The model under review builds one solid part; all positions refer to its coordinate system, in mm. A direction names the side the tool comes from. Coordinates: 2 decimals unless noted, no trailing zeros. Answer in a Markdown table with one row per item.
Autodesk Inventor part; units mm, degrees
ref_plane "YZ Plane" through (0, 0, 0) normal (1, 0, 0) x (0, 1, 0)
ref_plane "XZ Plane" through (0, 0, 0) normal (0, 1, 0) x (-1, 0, 0)
ref_plane "XY Plane" through (0, 0, 0) normal (0, 0, 1) x (1, 0, 0)
sketch "Sketch1" plane through (0, 0, 0) normal (0, 0, 1) x (1, 0, 0)
  line L0 (0, 0) -> (0, 24)
  line L1 (0, 24) -> (25, 24)
  line L2 (25, 24) -> (25, 4)
  line L3 (25, 4) -> (20, 4)
  line L4 (20, 4) -> (20, 0)
  line L5 (20, 0) -> (0, 0)
  line L6 (0, -4.8611) -> (0, 32.7303) construction
  dimension "d0" = 25
  dimension "d1" = 20
  dimension "d2" = 4
  dimension "d4" = 5
revolve "Revolution1" add sketch "Sketch1" angle 360 about axis through (0, -4.8611, 0) along (0, 1, 0)
sketch "Sketch9" plane through (0, 0, 0) normal (1, 0, 0) x (0, 1, 0)
  line L0 (0, 0) -> (-39.5663, 0) construction
  line L1 (4.5, -25) -> (5.5, -25)
  line L2 (5.5, -25) -> (5.5, -72.5)
  line L3 (5.5, -72.5) -> (4.5, -72.5)
  line L4 (4.5, -72.5) -> (4.5, -25)
  line L5 (0, -20) -> (0, 20)
  dimension "d28" = 1
  dimension "d29" = 25
  dimension "d30" = 4.5
  dimension "d31" = 47.5
coil "Coil1" sketch "Sketch9" operation add axis through (0, 0, 0) along (0, 1, 0) pitch 226 turns 0.077434 hand right
pattern_circular "Circular Pattern1" count 7 over 360 about axis through (0, 14, 0) along (0, 1, 0) of "Coil1"
equation "\"BendRadius\" = Thickness"
equation "\"BendReliefWidth\" = Thickness"
equation "\"BendReliefDepth\" = 0.5 * Thickness"
equation "\"CornerReliefSize\" = 4 * Thickness"
equation "\"MinimumRemnant\" = 2 * Thickness"
equation "\"TransitionRadius\" = BendRadius"
equation "\"JacobiRadiusSize\" = BendRadius"
equation "\"GapSize\" = Thickness"
properties part number "Ventoinha"
(1) Take a section at A-A (z = -36.5). State how many separate pieces and enclosed holes the cut face has, then the cut area to 3 significant figures.
Report:
| item | result |
|---|---|
| separate pieces | 3 |
| enclosed holes | 0 |
| area | 66.0 mm^2 |
(2) To check wall thickness, follow line 1 (X direction, y = 7, z = 38.5); line 2 (X direction, y = 9, z = 49); line 3 (Z direction, x = -34, y = 22.5). State the ranges of each line that lie inside material, in increasing order. Write a range as [from, to].
Report:
| item | result |
|---|---|
| line 1 | [-16.6, -15.35], [20.56, 21.96] |
| line 2 | [-17.97, -16.44], [29.78, 31.68] |
| line 3 | [-6.91, -6.42], [28.47, 29.28] |
(3) Insertion check: P1, Ø12, axis at x = -38.5, y = 3, coming from the +Z side; P2, Ø2, axis at x = -46.5, z = -13.5, coming from the -Y side; P3, Ø1.5, axis at x = -46.5, y = 19.5, coming from the -Z side. Each pin has a flat end and moves straight along its axis. Give the tip position at first contact, or say it passes through.
Report:
| item | result |
|---|---|
| P1 | z = 14.34 |
| P2 | y = 17.81 |
| P3 | z = -14.66 |
(4) The part is to be moulded in two halves that separate along X. For faces 4 (the flat face through (21.296, 4.993, 44.222)), 5 (the flat face through (-11, 4, -17)), 6 (the flat face through (-21.296, 4.993, 44.222)), say which applies: +X half, -X half, draft (parallel to the pull), parting line (faces both ways), or undercut.
Report:
| item | result |
|---|---|
| face 4 | undercut |
| face 5 | draft |
| face 6 | -X half |
(5) Machinability: for faces 1 (the flat face through (39.5, 22.49, 29.13)), 2 (the flat face through (-37.192, 22.493, 32.028)), 3 (the flat face through (-38.37, 4.99, -30.6)), which of the approach directions +Z, -Z, +X, -X, +Y, -Y give a long, thin tool a straight path to every point of the face, cutting with its end or side? Answer none if there is none.
Report:
| item | result |
|---|---|
| face 1 | +X, +Y, -Y |
| face 2 | +Z, +Y, -Y |
| face 3 | -Z, +Y, -Y |
